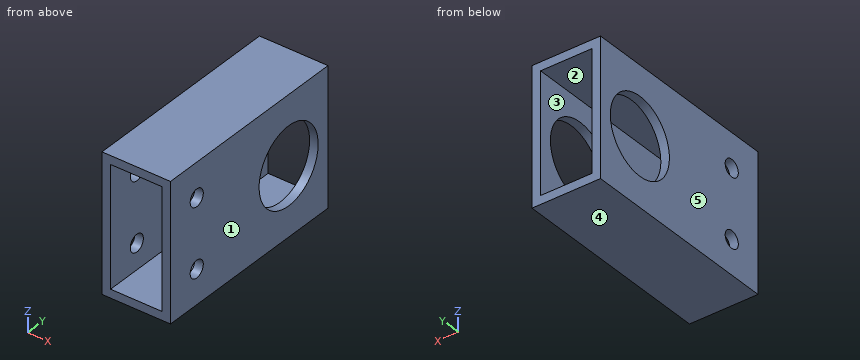
Autodesk Inventor part; units mm, degrees
ref_plane "YZ Plane" through (0, 0, 0) normal (1, 0, 0) x (0, 1, 0)
ref_plane "XZ Plane" through (0, 0, 0) normal (0, 1, 0) x (-1, 0, 0)
ref_plane "XY Plane" through (0, 0, 0) normal (0, 0, 1) x (1, 0, 0)
sketch "Sketch1" plane through (0, 0, 0) normal (0, 1, 0) x (-1, 0, 0)
  line L0 (0, 0) -> (25.4, 0)
  line L1 (25.4, 0) -> (25.4, -50.8)
  line L2 (25.4, -50.8) -> (0, -50.8)
  line L3 (0, -50.8) -> (0, 0)
  line L4 (22.225, -3.175) -> (3.175, -3.175)
  line L5 (3.175, -3.175) -> (3.175, -47.625)
  line L6 (3.175, -47.625) -> (22.225, -47.625)
  line L7 (22.225, -47.625) -> (22.225, -3.175)
  dimension "d0" = 50.8
  dimension "d1" = 25.4
  dimension "d2" = 3.175
  dimension "d3" = 3.175
  dimension "d4" = 3.175
  dimension "d5" = 3.175
extrude "Extrusion1" add sketch "Sketch1" along normal blind 76.2
sketch "Sketch2" plane through (0, 0, 0) normal (1, 0, 0) x (0, 0, -1)
  circle A0 centre (12.7, 12.7) radius 3.175
  circle A1 centre (38.1, 12.7) radius 3.175
  line L0 (50.8, 0) -> (0, 0)
  line L1 (0, 0) -> (0, 76.2)
  line L2 (50.8, 0) -> (50.8, 76.2)
  circle A2 centre (25.4, 57.15) radius 14.2875
  line L3 (0, 76.2) -> (50.8, 76.2)
  dimension "d8" = 12.7
  dimension "d9" = 6.35
  dimension "d10" = 12.7
  dimension "d11" = 12.7
  dimension "d12" = 12.7
  dimension "d13" = 6.35
  dimension "d14" = 28.575
  dimension "d15" = 19.05
  dimension "d16" = 25.4
extrude "Extrusion2" cut sketch "Sketch2" against normal blind 76.2 contours A0 | A1 | A2
equation "\"d3\" = d2"
equation "\"d4\" = d2"
equation "\"d5\" = d2"
properties part number "Hexshaft mount for 8020"
Design review of the part built by this model. Coordinates are the model's own, in mm. Face numbers are marked on the shaded views. A direction names the side the tool comes from. Coordinates: 2 decimals unless noted, no trailing zeros. Order: outer loops, then holes, each group sorted by start corner. A loop starts at its lowest first (then second) coordinate and runs counter-clockwise, first axis right, second up.
1) Take a section at B-B, the plane z = -25.4. Give the boundary of the cut face in (x, y) (1 decimal).
2) Mouldability with a two-part tool opening along Z and no side actions: class the marked faces 3, 4 and 5 as +Z half, -Z half, draft (parallel to the pull), parting line (faces both ways), or undercut.
3) For the marked faces 1 and 2, list the 3-axis set-ups (+Z, -Z, +X, -X, +Y, -Y) from which the entire face can be reached by the end or side of a thin tool; tool diameter is ignored.
4) Wall thickness on line 1 along X through (y, z) = (9.5, -14) (3 decimals); line 2 along Z through (x, y) = (-21, 36.5) (3 decimals); line 3 along Y through (x, z) = (-23, -12.7) (3 decimals): over which ranges is each line inside the solid? List them lowest first.
5) Take a section at D-D, the plane x = -8.5. Give the boundary of the cut face in (y, z) (3 decimals), and give its area (3 significant figures).
6) Take a section at A-A, the plane y = 57.15. Give the boundary of the cut face in (x, z) (1 decimal), and give its area (3 significant figures).
7) Take a section at C-C, the plane y = 12.7. Give the boundary of the cut face in (x, z) (3 decimals).
Returned:
1. outline: (-25.4, 0) - (-22.2, 0) - (-22.2, 42.9) - (-25.4, 42.9) - close; (-25.4, 71.4) - (-22.2, 71.4) - (-22.2, 76.2) - (-25.4, 76.2) - close; (-3.2, 0) - (0, 0) - (0, 42.9) - (-3.2, 42.9) - close; (-3.2, 71.4) - (0, 71.4) - (0, 76.2) - (-3.2, 76.2) - close
2. face 3: undercut
2. face 4: -Z half
2. face 5: draft
3. face 1: +Z, -Z, +X, +Y, -Y
3. face 2: +Y, -Y
4. line 1: x = -25.4 to -22.225, -3.175 to 0
4. line 2: z = -50.8 to -47.625, -3.175 to 0
4. line 3: y = 0 to 9.525, 15.875 to 50.605, 63.695 to 76.2
5. outline: (0, -50.8) - (76.2, -50.8) - (76.2, -47.625) - (0, -47.625) - close; (0, -3.175) - (76.2, -3.175) - (76.2, 0) - (0, 0) - close
5. area: 484 mm2
6. outline: (-25.4, -50.8) - (0, -50.8) - (0, -39.7) - (-3.2, -39.7) - (-3.2, -47.6) - (-22.2, -47.6) - (-22.2, -39.7) - (-25.4, -39.7) - close; (-25.4, -11.1) - (-22.2, -11.1) - (-22.2, -3.2) - (-3.2, -3.2) - (-3.2, -11.1) - (0, -11.1) - (0, 0) - (-25.4, 0) - close
6. area: 262 mm2
7. outline: (-25.4, -50.8) - (0, -50.8) - (0, -41.275) - (-3.175, -41.275) - (-3.175, -47.625) - (-22.225, -47.625) - (-22.225, -41.275) - (-25.4, -41.275) - close; (-25.4, -34.925) - (-22.225, -34.925) - (-22.225, -15.875) - (-25.4, -15.875) - close; (-25.4, -9.525) - (-22.225, -9.525) - (-22.225, -3.175) - (-3.175, -3.175) - (-3.175, -9.525) - (0, -9.525) - (0, 0) - (-25.4, 0) - close; (-3.175, -34.925) - (0, -34.925) - (0, -15.875) - (-3.175, -15.875) - close
